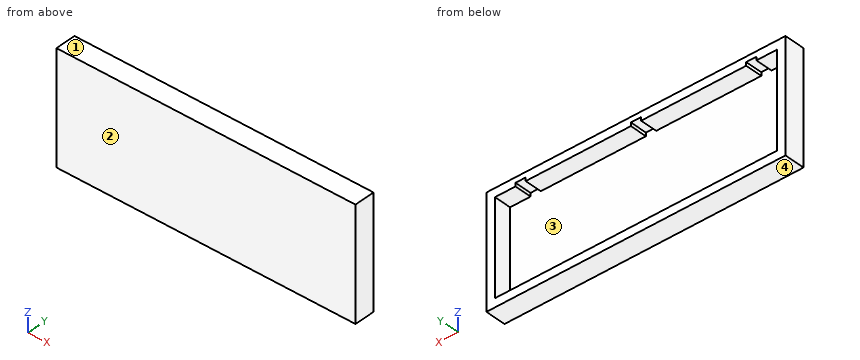
```python
from build123d import *

# Parameters (mm, degrees)
SKETCH1_W           = 175
SKETCH1_H           = 65
BOSS_EXTRUDE1_DEPTH = 12
SKETCH2_W           = 165
SKETCH2_H           = 55
CUT_EXTRUDE1_DEPTH  = 10
SKETCH5_W           = 6
SKETCH5_H           = 10
CUT_EXTRUDE2_DEPTH  = 2
SKETCH6_W           = 6
SKETCH6_H           = 10
CUT_EXTRUDE3_DEPTH  = 2
SKETCH7_W           = 6
SKETCH7_H           = 10
CUT_EXTRUDE4_DEPTH  = 2


with BuildPart() as part:
    # Sketch1 → Boss-Extrude1 (new body)
    with BuildSketch(Plane(origin=(0, 0, 0), x_dir=(1, 0, 0), z_dir=(0, 1, 0))):
        Rectangle(SKETCH1_W, SKETCH1_H)
    extrude(amount=BOSS_EXTRUDE1_DEPTH)

    # Sketch2 → Cut-Extrude1 (cut)
    with BuildSketch(Plane(origin=(0, 12, 0), x_dir=(1, 0, 0), z_dir=(0, 1, 0))):
        Rectangle(SKETCH2_W, SKETCH2_H)
    extrude(amount=-CUT_EXTRUDE1_DEPTH, mode=Mode.SUBTRACT)

    # Sketch5 → Cut-Extrude2 (cut)
    with BuildSketch(Plane(origin=(0, 0, 27.5), x_dir=(-1, 0, 0), z_dir=(0, 0, -1))):
        with Locations((0, 7)):
            Rectangle(SKETCH5_W, SKETCH5_H)
    extrude(amount=-CUT_EXTRUDE2_DEPTH, mode=Mode.SUBTRACT)

    # Sketch6 → Cut-Extrude3 (cut)
    with BuildSketch(Plane(origin=(0, 0, 27.5), x_dir=(-1, 0, 0), z_dir=(0, 0, -1))):
        with Locations((-67.5, 7)):
            Rectangle(SKETCH6_W, SKETCH6_H)
    extrude(amount=-CUT_EXTRUDE3_DEPTH, mode=Mode.SUBTRACT)

    # Sketch7 → Cut-Extrude4 (cut)
    with BuildSketch(Plane(origin=(0, 0, 27.5), x_dir=(-1, 0, 0), z_dir=(0, 0, -1))):
        with Locations((67.5, 7)):
            Rectangle(SKETCH7_W, SKETCH7_H)
    extrude(amount=-CUT_EXTRUDE4_DEPTH, mode=Mode.SUBTRACT)


solid = part.part
```
Here's how the part is built. I have some questions about the finished solid (model axes, mm). Face numbers are marked on the shaded views. Round coordinates to 2 decimals unless told otherwise and drop trailing zeros. Loops run counter-clockwise (first coordinate to the right, second up) from the corner with the lowest first, then second, coordinate; pieces in that order, holes last. Notation, with made-up numbers: (9, 10) -> (19, 10) arc R20 ccw to (19, 29) -> close; hole circle Ø1 at (20, 13). An arc over 180 degrees is marked (long way). Answer as CSV lines item,"result". Start each with the question number.
1. I'm going to push a flat-ended pin straight in: P1, Ø12, axis at x = -37, z = -0.5, coming from the +Y side. Where does the tip first touch, or does it pass through?
2. Imagine slicing it at B-B on x = -26. Write out the boundary of the cut face in (y, z).
3. I need wall thicknesses on probe 1 along Z at (x, y) = (-72.5, 5.25); probe 2 along X at (y, z) = (2.5, 7.5); probe 3 along Z at (x, y) = (-2, 6.25). Which ranges of each line are inside material? Lowest first, please. Write a range as from..to.
4. Imagine slicing it at A-A on y = 5.75. Write out the boundary of the cut face in (x, z).
5. If we mould it in two halves opening along Z, with no side actions, what happens to the marked faces 1, 2, 3 and 4? For each: pulls with the +Z half, pulls with the -Z half, needs draft (parallel to the pull), parting line crosses it, or undercut.
6. Imagine slicing it at C-C on z = -5. Write out the boundary of the cut face in (x, y), plus the area to 3 significant figures.
Solution:
1,P1,"y = 2"
2,outline,"(0, -32.5) -> (12, -32.5) -> (12, -27.5) -> (2, -27.5) -> (2, 27.5) -> (12, 27.5) -> (12, 32.5) -> (0, 32.5) -> close"
3,probe 1,"-32.5..-27.5, 27.5..32.5"
3,probe 2,"-87.5..-82.5, 82.5..87.5"
3,probe 3,"-32.5..-27.5, 29.5..32.5"
4,outline,"(-87.5, -32.5) -> (87.5, -32.5) -> (87.5, 32.5) -> (-87.5, 32.5) -> close; hole (-82.5, -27.5) -> (82.5, -27.5) -> (82.5, 27.5) -> (70.5, 27.5) -> (70.5, 29.5) -> (64.5, 29.5) -> (64.5, 27.5) -> (3, 27.5) -> (3, 29.5) -> (-3, 29.5) -> (-3, 27.5) -> (-64.5, 27.5) -> (-64.5, 29.5) -> (-70.5, 29.5) -> (-70.5, 27.5) -> (-82.5, 27.5) -> close"
5,face 1,"pulls with the +Z half"
5,face 2,"needs draft"
5,face 3,"undercut"
5,face 4,"pulls with the -Z half"
6,outline,"(-87.5, 0) -> (87.5, 0) -> (87.5, 12) -> (82.5, 12) -> (82.5, 2) -> (-82.5, 2) -> (-82.5, 12) -> (-87.5, 12) -> close"
6,area,"450 mm²"
